For this review, take the finished solid that the model builds, in its own axes (mm). Face numbers are marked on the shaded views. A direction names the side the tool comes from. Coordinates: 2 decimals unless noted, no trailing zeros. Write each loop counter-clockwise with the first axis right and the second up, starting at its lowest first coordinate (ties: lowest second). Pieces come first, ordered by that corner, then holes.
```python
from build123d import *

# Parameters (mm, degrees)
F1_DEPTH    = 3.175
F2_START    = 3.048
F2_DEPTH    = 530.352
F3_T        = 2.54
F3_T3_DEPTH = 8.128
F3_T5_DEPTH = 220.6061469057
F3_T7_DEPTH = 239.2564292152
F3_T9_DEPTH = 462.28
F5_DEPTH    = 3.175


# Not quite as in the source:
# - a shell that OpenCascade refuses in one call is made with other operations: the cavity is built on its own and cut out


with BuildPart() as f1:
    # F0 (on Front) → F1 (new body)
    with BuildSketch(Plane.XZ):
        Polygon((-63.5, 0), (0, 0), (0, 254), (-914.4, 254), (-914.4, 0), (-850.9, 0), (-673.1, 152.4), (-215.9, 152.4), align=None)
    extrude(amount=F1_DEPTH)

    # F0 (on Front) → F2 (join)
    with BuildSketch(Plane.XZ.offset(F2_START)):
        Polygon((-850.9, 0), (-63.5, 0), (-215.9, 152.4), (-673.1, 152.4), align=None)
    extrude(amount=F2_DEPTH)

    # F3: shell of thickness 2.54, made by hand


with BuildPart() as f3_core1:
    # F3_t2: copy of F1
    add(f1.part)

    # the walls: a layer under each face that stays
    f3_faces = [f3_core1.faces().sort_by_distance(p)[0] for p in [
        (-139.7, -1.524, 76.2),
        (-762, 0, 127),
        (-444.5, -1.524, 152.4),
        (0, -1.5875, 127),
        (-457.2, -1.5875, 254),
        (-914.4, -1.5875, 127),
        (-762, -1.524, 76.2),
        (-762, -3.175, 127),
        (-762, -268.2875, 76.2),
        (-139.7, -268.2875, 76.2),
        (-457.2, -533.4, 76.2),
        (-444.5, -268.2875, 152.4),
    ]]
    thicken(f3_faces, amount=-F3_T, mode=Mode.SUBTRACT)

    # F3_s4 → F3_t3 (cut)
    with BuildSketch(Plane.XZ.offset(-2.54)):
        Polygon((-215.9179605122, 152.3566394878), (-214.1039487758, 154.1960512242), (-214.8478975516, 154.94), (-215.9, 154.94), align=None)
        Polygon((-673.0834698991, 152.3553148823), (-673.1, 154.94), (-674.0396071536, 154.94), (-674.7530100886, 154.32851177), align=None)
    extrude(amount=F3_T3_DEPTH, mode=Mode.SUBTRACT)

    # F3_s6 → F3_t5 (cut)
    with BuildSketch(Plane(origin=(-185.9460512242, 0, 185.9460512242), x_dir=(0, 1, 0), z_dir=(0.7071067812, 0, -0.7071067812))):
        Polygon((-3.2004, -44.8758806053), (-0.635, -44.9012806053), (-0.635, -47.4412806053), (-3.175, -47.4412806053), align=None)
    extrude(amount=F3_T5_DEPTH, mode=Mode.SUBTRACT)

    # F3_s8 → F3_t7 (cut)
    with BuildSketch(Plane(origin=(-492.4473352994, 0, -422.0977159709), x_dir=(0, 1, 0), z_dir=(0.7592566024, 0, 0.6507913735))):
        Polygon((-3.2004, 553.7837796737), (-0.635, 553.7583796737), (-0.635, 551.2183796737), (-3.175, 551.2183796737), align=None)
    extrude(amount=F3_T7_DEPTH, mode=Mode.SUBTRACT)

    # F3_s10 → F3_t9 (cut)
    with BuildSketch(Plane.YZ.offset(-675.64)):
        Polygon((-3.2004, 152.4254), (-0.635, 152.4), (-0.635, 149.86), (-3.175, 149.86), align=None)
    extrude(amount=F3_T9_DEPTH, mode=Mode.SUBTRACT)


with BuildPart() as f1_1:
    add(f1.part)

    # what is left inside the walls is the cavity
    f3_cavity = [f3_core1.part.solids().sort_by_distance(p)[0] for p in [
        (-457.044581, -354.922667, 0.0254),
    ]]
    add(f3_cavity, mode=Mode.SUBTRACT)

    # F4 (on Top) → F5 (join)
    with BuildSketch(Plane.XY):
        Polygon((0, -558.8), (0, 0), (-69.1089183092, 0), (-69.1089183092, -530.9250950813), (-844.7285890579, -530.9250950813), (-844.7285890579, 0), (-916.9259883143, 0), (-916.9259883143, -558.8), align=None)
    extrude(amount=F5_DEPTH)


solid = f1_1.part
```
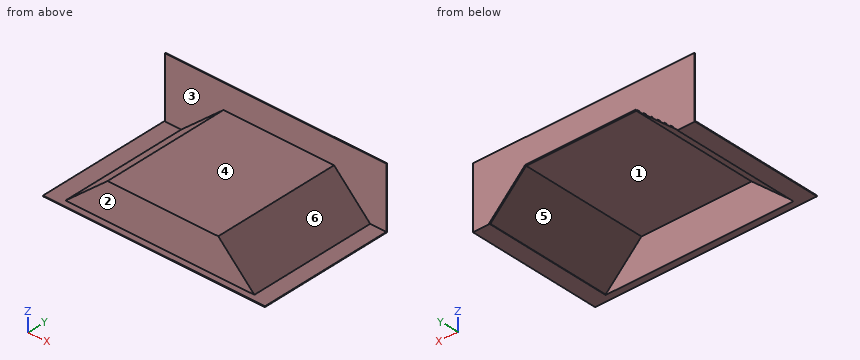
Q1. Tool access review of the marked faces 1, 2 and 3: name each direction out of +Z, -Z, +X, -X, +Y, -Y from which nothing blocks a thin tool from reaching the whole face with its end or side.
Ans:
face 1: -Z, +Y
face 2: +Z, +X, -X, -Y
face 3: +Z, -Y
Q2. Add section C-C (z = 53.5). State the section outline as (x, y) points (3 decimals).
Ans:
outline: (-914.4, -3.175) - (-788.483, -3.175) - (-788.483, -533.4) - (-117, -533.4) - (-117, -3.175) - (0, -3.175) - (0, 0) - (-117, 0) - (-117, -3.048) - (-120.592, -3.048) - (-120.592, -530.86) - (-784.58, -530.86) - (-784.58, -3.048) - (-788.483, -3.048) - (-788.483, 0) - (-914.4, 0) - close
Q3. Add section B-B (y = -492.5). State the section outline as (x, z) points (3 decimals).
Ans:
outline: (-916.926, 0) - (-844.729, 0) - (-844.729, 1.944) - (-672.16, 149.86) - (-216.952, 149.86) - (-69.109, 2.017) - (-69.109, 0) - (0, 0) - (0, 3.175) - (-66.675, 3.175) - (-215.9, 152.4) - (-673.1, 152.4) - (-847.196, 3.175) - (-916.926, 3.175) - close
Q4. Clearance check with flat-ended pins moving along their axes: pin 1 Ø8 at (x, y) = (-314, -449) entering from +Z; pin 2 Ø2.5 at (x, y) = (-391, -1) entering from -Z; pin 3 Ø6 at (y, z) = (-283.5, 122) entering from -X. State where each tip first meets the part, or that it passes through.
Ans:
pin 1: stops at z = 152.4
pin 2: stops at z = 152.4
pin 3: stops at x = -712.07
Q5. For probe 1 along Y at (x, z) = (-603, 159) (3 decimals); probe 2 along Y at (x, z) = (-234, 12); probe 3 along Z at (x, y) = (-277.5, -444), list the stretches that pass through material, from the lowest coordinate up.
Ans:
probe 1: y = -3.175 to 0
probe 2: y = -533.4 to -530.86
probe 3: z = 149.86 to 152.4
Q6. Draft analysis for pull direction X (two halves, no side actions). For the marked faces 4, 5 and 6, state which applies: +X half, -X half, draft (parallel to the pull), parting line (faces both ways), or undercut.
Ans:
face 4: draft
face 5: undercut
face 6: +X half
Q7. Add section D-D (x = -861). State the section outline as (y, z) points (3 decimals).
Ans:
outline: (-558.8, 0) - (0, 0) - (0, 254) - (-3.175, 254) - (-3.175, 3.175) - (-558.8, 3.175) - close
Q8. Add section A-A (x = -244). State the section outline as (y, z) points (3 decimals).
Ans:
outline: (-558.8, 0) - (-530.86, 0) - (-530.86, 149.86) - (-3.048, 149.86) - (-3.048, 152.4) - (0, 152.4) - (0, 254) - (-3.175, 254) - (-3.175, 152.4) - (-533.4, 152.4) - (-533.4, 3.175) - (-558.8, 3.175) - close
